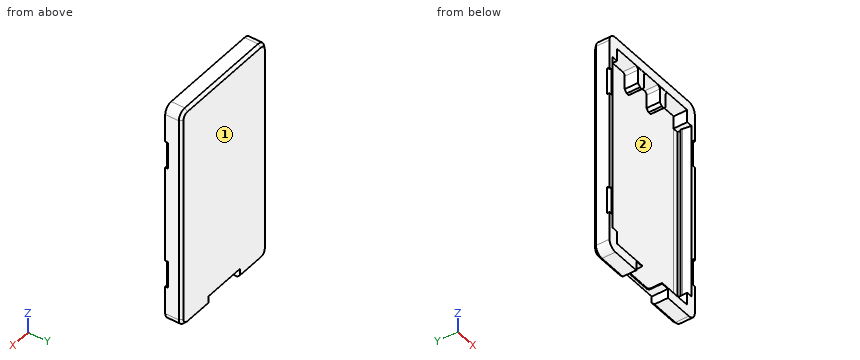
Autodesk Inventor part; units mm, degrees
ref_plane "Work Plane3" through (-17.7, 0, 76.2) normal (1, 0, 0) x (0, 0, -1)
ref_plane "Work Plane4" through (0.8, 0, 65.7) normal (0, 0, -1) x (-1, 0, 0)
ref_plane "YZ Plane" through (0, 0, 0) normal (1, 0, 0) x (0, 1, 0)
sketch "Sketch1" plane through (0, 0, 0) normal (0, 1, 0) x (-1, 0, 0)
  line L0 (0, 0) -> (35.4, 0)
  line L1 (35.4, 0) -> (35.4, 75.4)
  line L2 (35.4, 75.4) -> (0, 75.4)
  line L3 (0, 75.4) -> (0, 0)
  line L4 (39.2, -3.8) -> (-3.8, -3.8)
  line L5 (-3.8, -3.8) -> (-3.8, 79.2)
  line L6 (-3.8, 79.2) -> (39.2, 79.2)
  line L7 (39.2, 79.2) -> (39.2, -3.8)
  line L8 (39.2, 37.7) -> (49.7975, 37.7) construction
  line L9 (17.7, 79.2) -> (17.7, 95.7522) construction
  line L10 (24.7, 75.4) -> (21.7, 75.4)
  line L11 (21.7, 75.4) -> (21.7, 68.4)
  line L12 (21.7, 68.4) -> (24.7, 68.4)
  line L13 (24.7, 68.4) -> (24.7, 75.4)
  line L14 (13.7, 75.4) -> (10.7, 75.4)
  line L15 (10.7, 75.4) -> (10.7, 68.4)
  line L16 (10.7, 68.4) -> (13.7, 68.4)
  line L17 (13.7, 68.4) -> (13.7, 75.4)
  line L18 (0.2, 75.2) -> (35.2, 75.2)
  line L19 (35.2, 75.2) -> (35.2, 0.2)
  line L20 (35.2, 0.2) -> (0.2, 0.2)
  line L21 (0.2, 0.2) -> (0.2, 75.2)
  point P0 (21.7, 75.4)
  point P1 (10.7, 75.4)
  dimension "d43" = 4
  dimension "d44" = 4
  dimension "d45" = 7
  dimension "d46" = 3
  dimension "d47" = 3
  dimension "d74" = 0.2
  dimension "d75" = 75
  dimension "d76" = 35
  dimension "d77" = 4
extrude "Extrusion1" add sketch "Sketch1" along normal blind 6 contours L3 L2 L15 L18 L21 L20 L19 L13 L1 L0 | L2 L17 L18 L15 | L13 L18 L11 L2 | L2 L11 L18 L17 | L18 L17 L16 L15 | L15 L16 L17 L18 L11 L12 L13 L19 L20 L21 | L13 L12 L11 L18 | L4 L5 L6 L7
extrude "Extrusion2" cut sketch "Sketch1" along normal blind 5 contours L3 L2 L15 L18 L21 L20 L19 L13 L1 L0 | L2 L11 L18 L17 | L15 L16 L17 L18 L11 L12 L13 L19 L20 L21
sketch "Sketch3" plane through (5, 0, -3.8) normal (0, 0, -1) x (-1, 0, 0)
  line L0 (22.7, 10) -> (22.7, 15.0736) construction
  line L1 (29.7, 8) -> (15.7, 8)
  line L2 (14.7, 7) -> (14.7, 0)
  line L3 (30.7, 0) -> (30.7, 7)
  arc A0 (30.7, 7) -> (29.7, 8) centre (29.7, 7) ccw
  arc A1 (15.7, 8) -> (14.7, 7) centre (15.7, 7) ccw
  line L4 (30.7, 0) -> (14.7, 0)
  line L5 (1.2, 0) -> (44.2, 0)
  line L6 (44.2, 0) -> (1.2, 0)
  line L7 (17.7, 0) -> (17.7, 4.1)
  line L8 (18.7, 5.1) -> (26.7, 5.1)
  line L9 (27.7, 4.1) -> (27.7, 0)
  arc A2 (18.7, 5.1) -> (17.7, 4.1) centre (18.7, 4.1) ccw
  arc A3 (27.7, 4.1) -> (26.7, 5.1) centre (26.7, 4.1) ccw
  line L10 (1.2, 0) -> (1.2, 6)
  line L11 (44.2, 0) -> (44.2, 6)
  point P0 (30.5, 8)
  point P1 (14.5, 8)
  point P2 (17.7, 0)
  dimension "d15" = 8
  dimension "d16" = 8
  dimension "d19" = 1
  dimension "d27" = 5.1
  dimension "d28" = 5
  dimension "d29" = 5
  dimension "d30" = 1
  dimension "d33" = 21.5
  dimension "d34" = 43
  dimension "d35" = 8
extrude "Extrusion3" cut sketch "Sketch3" against normal up to surface (3.8 mm away) contours L4 L7 A2 L8 A3 L9
extrude "Extrusion4" cut sketch "Sketch3" against normal blind 3.5 contours A0 L3 L4 L9 A3 L8 A2 L7 L2 A1 L1
fillet "Fillet1" radius 3 4 edges at (3.8, 3, -3.8) (-39.2, 3, -3.8) (3.8, 3, 79.2) (-39.2, 3, 79.2)
chamfer "Chamfer3" distance 1 angle 45 9 edges at (-30.95, 6, -3.8) (-4.45, 6, -3.8) (-38.3213, 6, -2.9213) (-39.2, 6, 37.7) (-38.3213, 6, 78.3213) (-17.7, 6, 79.2) (2.9213, 6, 78.3213) (3.8, 6, 37.7) (2.9213, 6, -2.9213)
fillet "Fillet2" radius 1 4 edges at (-24.7, 2.5, 75.4) (-21.7, 2.5, 75.4) (-13.7, 2.5, 75.4) (-10.7, 2.5, 75.4)
chamfer "Chamfer5" distance 1 angle 45 4 edges at (-24.7, 2.5, 68.4) (-21.7, 2.5, 68.4) (-13.7, 2.5, 68.4) (-10.7, 2.5, 68.4)
ref_plane "Work Plane2" through (0.8, 0, 67.7) normal (0, 0, -1) x (-1, 0, 0)
ref_plane "Work Plane1" through (0.8, 0, 37.7) normal (0, 0, -1) x (-1, 0, 0)
ref_plane "Work Plane3" through (-17.7, 0, 76.2) normal (1, 0, 0) x (0, 0, -1)
ref_plane "Work Plane4" through (0.8, 0, 65.7) normal (0, 0, -1) x (-1, 0, 0)
sketch "Sketch4" plane through (0.8, 0, 37.7) normal (0, 0, -1) x (-1, 0, 0)
  line L0 (36.2, 0) -> (36.2, 5)
  line L1 (36.2, 0) -> (37.8, 0) construction
  line L2 (40, 0) -> (36.2, 0)
  line L3 (37.8, 0) -> (37.8, 5) construction
  line L4 (38.15, 4.65) -> (38.15, 3.9) construction
  line L5 (37.8, 5) -> (36.2, 5) construction
  line L6 (37.8, 5) -> (38.15, 4.65) construction
  line L7 (38.15, 3.9) -> (37.8, 3.55) construction
  line L8 (38.4, 0) -> (37.9, 3)
  line L9 (37.9, 3) -> (37.9, 3.65)
  line L10 (37.9, 3.65) -> (38.25, 4)
  line L11 (38.25, 4) -> (38.25, 5.1)
  line L12 (36.2, 0) -> (0.8, 0)
  line L13 (38.4, 0) -> (36.2, 0)
  line L14 (36.2, 0) -> (36.2, 5)
  line L15 (38.25, 5.1) -> (36.2, 5.1)
  line L16 (36.2, 5.1) -> (36.2, 5)
  line L17 (37, 0) -> (37, 5)
  line L18 (36.2, 5.1) -> (36.1, 5)
  line L19 (36.2, 5) -> (26.5, 5)
  line L20 (36.2, 5) -> (36.1, 5)
  dimension "d53" = 1.6
  dimension "d54" = 5
  dimension "d55" = 0.35
  dimension "d58" = 45
  dimension "d59" = 45
  dimension "d60" = 1.1
  dimension "d61" = 0.1
  dimension "d62" = 0.6
  dimension "d63" = 3
  dimension "d64" = 0.1
  dimension "d83" = 135
  dimension "d84" = 0.1
sketch "Sketch5" plane through (0.8, 0, 67.7) normal (0, 0, -1) x (-1, 0, 0)
  line L0 (40, 5) -> (40, 0)
  line L1 (40, 1) -> (39, 0)
  line L2 (40, 0) -> (37, 0)
  line L3 (40, 1) -> (40, 0)
  line L4 (39, 0) -> (40, 0)
  point P0 (0.8, 0)
  dimension "d65" = 45
  dimension "d66" = 1
extrude "Extrusion5" cut sketch "Sketch5" along normal blind 10 from surface at 2
extrude "Extrusion6" cut sketch "Sketch4" against normal blind 33 and the other way blind 3.5
mirror "Mirror1" about plane through (0.8, 0, 37.7) normal (0, 0, -1) of "Extrusion6", "Extrusion5"
mirror "Mirror2" about plane through (-17.7, 0, 76.2) normal (1, 0, 0) of "Extrusion6", "Extrusion5", "Mirror1"
extrude "Extrusion7" cut sketch "Sketch1" along normal blind 0.1 contours L3 L2 L15 L18 L21 L20 L19 L13 L1 L0 | L2 L17 L18 L15 | L13 L18 L11 L2 | L2 L11 L18 L17 | L18 L17 L16 L15 | L15 L16 L17 L18 L11 L12 L13 L19 L20 L21 | L13 L12 L11 L18
equation "\"d43\" = d44"
equation "\"d47\" = d46"
equation "\"d16\" = d15"
equation "\"d29\" = d28"
equation "\"d33\" = 0.5 * d34"
properties part number "scatola_v2_sopra"
Model file for the job. Use its own axes, mm. Face numbers are marked on the shaded views. A direction names the side the tool comes from. Coordinates: 2 decimals unless noted, no trailing zeros. Write each loop counter-clockwise with the first axis right and the second up, starting at its lowest first coordinate (ties: lowest second). Pieces come first, ordered by that corner, then holes. Notation, with made-up numbers: (69.25, 62) -> (102.25, 62) arc R12 ccw to (102.25, 84) -> close; hole circle Ø4 at (83.5, 6). An arc over 180 degrees is marked (long way). One line per item, written item: value. Start each with the question number.
1) Slice it at D-D on x = -7. Write the cut outline in (y, z).
2) Slice it at C-C on z = 58.5. Write the cut outline in (x, y), then the cut area to 3 significant figures.
3) Flat gauge pins, fed straight in: pin 1 Ø10 at (x, z) = (-33, 56) entering from -Y; pin 2 Ø0.5 at (x, y) = (-38.5, 0.5) entering from -Z; pin 3 Ø4 at (x, z) = (-11, 72.5) entering from -Y; pin 4 Ø0.8 at (x, y) = (3, 0.5) entering from +Z. Where does each tip first touch, or does it go through?
4) Which spindle directions (+Z, -Z, +X, -X, +Y, -Y) get a long thin tool onto all of the face, cutting with end or side? Do the marked faces 1 and 2. Say none if no direction does.
5) Slice it at B-B on x = -19. Write the cut outline in (y, z), then the cut area to 3 significant figures.
6) Probe probe 1 along X at (y, z) = (2.5, 73); probe 2 along X at (y, z) = (4.2, 39); probe 3 along Z at (x, y) = (-6, 4.9). List the from-to ranges inside material, lowest first.
7) Slice it at A-A on z = 2. Write the cut outline in (x, y).
Answers follow:
1. outline: (0, -3.8) -> (5, -3.8) -> (6, -2.8) -> (6, 78.2) -> (5, 79.2) -> (0, 79.2) -> (0, 75.4) -> (5, 75.4) -> (5, 0) -> (0, 0) -> close
2. outline: (-39.2, 1) -> (-38.2, 0) -> (-37.6, 0) -> (-37.1, 3) -> (-37.1, 3.65) -> (-37.45, 4) -> (-37.45, 5.1) -> (-35.4, 5.1) -> (-35.3, 5) -> (-0.1, 5) -> (0, 5.1) -> (2.05, 5.1) -> (2.05, 4) -> (1.7, 3.65) -> (1.7, 3) -> (2.2, 0) -> (2.8, 0) -> (3.8, 1) -> (3.8, 5) -> (2.8, 6) -> (-38.2, 6) -> (-39.2, 5) -> close
2. area: 59.3 mm2
3. pin 1: y = 0
3. pin 2: z = -2.99
3. pin 3: y = 0.1
3. pin 4: z = 78.6
4. face 1: +Z, -Z, +X, -X, +Y
4. face 2: -Y
5. outline: (0, 75.4) -> (5, 75.4) -> (5, 0) -> (5.1, 0) -> (5.1, -0.3) -> (6, -0.3) -> (6, 78.2) -> (5, 79.2) -> (0, 79.2) -> close
5. area: 98.0 mm2
6. probe 1: -39.2 to -35.4, -24.7 to -21.7, -13.7 to -10.7, 0 to 3.8
6. probe 2: -39.2 to -37.45, 2.05 to 3.8
6. probe 3: -3.8 to 0, 75.4 to 79.2
7. outline: (-39.2, 0) -> (-35.4, 0) -> (-35.4, 5) -> (0, 5) -> (0, 0) -> (3.8, 0) -> (3.8, 5) -> (2.8, 6) -> (-38.2, 6) -> (-39.2, 5) -> close
